The drawing under review shows one solid part. Ordinate dimensions are in mm from its lowest x, y, z. A direction names the side the tool comes from. Coordinates: 2 decimals unless noted, no trailing zeros. Write each loop counter-clockwise with the first axis right and the second up, starting at its lowest first coordinate (ties: lowest second). Pieces come first, ordered by that corner, then holes.
Q1. Insertion check: pin 1 (8 mm diameter, centred on x = 25, y = 15, fed in from -Z); pin 2 (6 mm diameter, centred on y = 15.5, z = 48.5, fed in from +X); pin 3 (5 mm diameter, centred on y = 9, z = 10, fed in from -X); pin 4 (4 mm diameter, centred on x = 18.5, z = 62, fed in from +Y). Each pin has a flat end and moves straight along its axis. Give the tip position at first contact, or say it passes through.
Q2. Take a section at B-B (z = 48). Give the boundary of the cut face in (x, y), and give its area (3 significant figures).
Q3. Machinability: for the marked faces 1, 2 and 3, which of the approach directions +Z, -Z, +X, -X, +Y, -Y give a long, thin tool a straight path to every point of the face, cutting with its end or side? Answer none if there is none.
Q4. Take a section at C-C (x = 25.5). Give the boundary of the cut face in (y, z).
Q5. For probe 1 along Z at (x, y) = (20, 2); probe 2 along Y at (x, z) = (18, 31.5); probe 3 along Z at (x, y) = (4, 28), list the stretches that pass through material, from the lowest coordinate up.
Q6. Take a section at A-A (y = 18.5). Give the boundary of the cut face in (x, z).
Q7. Take a section at D-D (y = 11.15). Give the boundary of the cut face in (x, z), and give its area (3 significant figures).
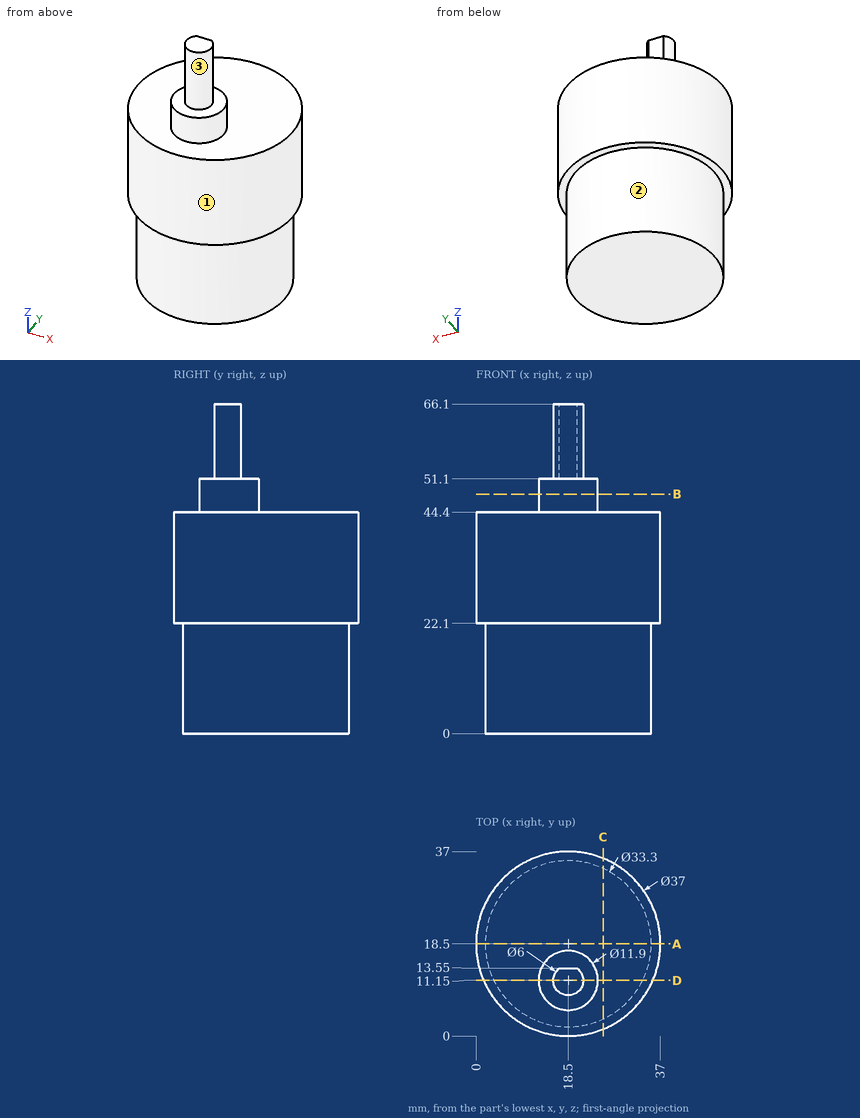
Response:
1. pin 1: stops at z = 0
1. pin 2: stops at x = 24.29
1. pin 3: stops at x = 3.39
1. pin 4: stops at y = 13.55
2. outline: circle Ø11.9 at (18.5, 11.15)
2. area: 111 mm2
3. face 1: +Z, -Z
3. face 2: -Z
3. face 3: +Z
4. outline: (1.38, 22.1) - (3.39, 22.1) - (3.39, 0) - (33.61, 0) - (33.61, 22.1) - (35.62, 22.1) - (35.62, 44.4) - (1.38, 44.4) - close
5. probe 1: z = 0 to 44.4
5. probe 2: y = 0.01 to 36.99
5. probe 3: z = 22.1 to 44.4
6. outline: (0, 22.1) - (1.85, 22.1) - (1.85, 0) - (35.15, 0) - (35.15, 22.1) - (37, 22.1) - (37, 44.4) - (0, 44.4) - close
7. outline: (1.52, 22.1) - (3.56, 22.1) - (3.56, 0) - (33.44, 0) - (33.44, 22.1) - (35.48, 22.1) - (35.48, 44.4) - (24.45, 44.4) - (24.45, 51.1) - (21.5, 51.1) - (21.5, 66.1) - (15.5, 66.1) - (15.5, 51.1) - (12.55, 51.1) - (12.55, 44.4) - (1.52, 44.4) - close
7. area: 1,590 mm2
